For this review, use the dimensioned drawing (mm, ordinates from the lowest corner) and the shaded views. A direction names the side the tool comes from. Round coordinates to 2 decimals unless told otherwise and drop trailing zeros. Order: outer loops, then holes, each group sorted by start corner. A loop starts at its lowest first (then second) coordinate and runs counter-clockwise, first axis right, second up. Notation, with made-up numbers: (-29.5, 18.25) - (-1.5, 18.25) arc R14 ccw to (-1.5, 29.25) - close; hole circle Ø6 at (-29, 80). An arc over 180 degrees is marked (long way). Write each question's results on one line, items separated by ' | '. Start each with the question number.
(1) For the marked faces 1 and 2, list the 3-axis set-ups (+Z, -Z, +X, -X, +Y, -Y) from which the entire face can be reached by the end or side of a thin tool; tool diameter is ignored.
(2) Draft analysis for pull direction X (two halves, no side actions). For the marked faces 3, 4 and 5, state which applies: pulls with the +X half, pulls with the -X half, needs draft (parallel to the pull), parting line crosses it, or undercut.
(3) Take a section at C-C, the plane x = 482.55. Give the boundary of the cut face in (y, z), plus the area to 3 significant figures.
(4) Take a section at A-A, the plane y = 286.5. Give the boundary of the cut face in (x, z).
(5) Take a section at D-D, the plane y = 484. Give the boundary of the cut face in (x, z).
(6) Take a section at B-B, the plane z = 54. Give the boundary of the cut face in (x, y), plus the area to 3 significant figures.
(7) For L1, parallel to X at y = 526, z = 31; L2, parallel to X at y = 282.5, z = 18; L3, parallel to Y at x = 495, z = 94.5, list the stretches that pass through material, from the lowest coordinate up. Write a range as from..to.
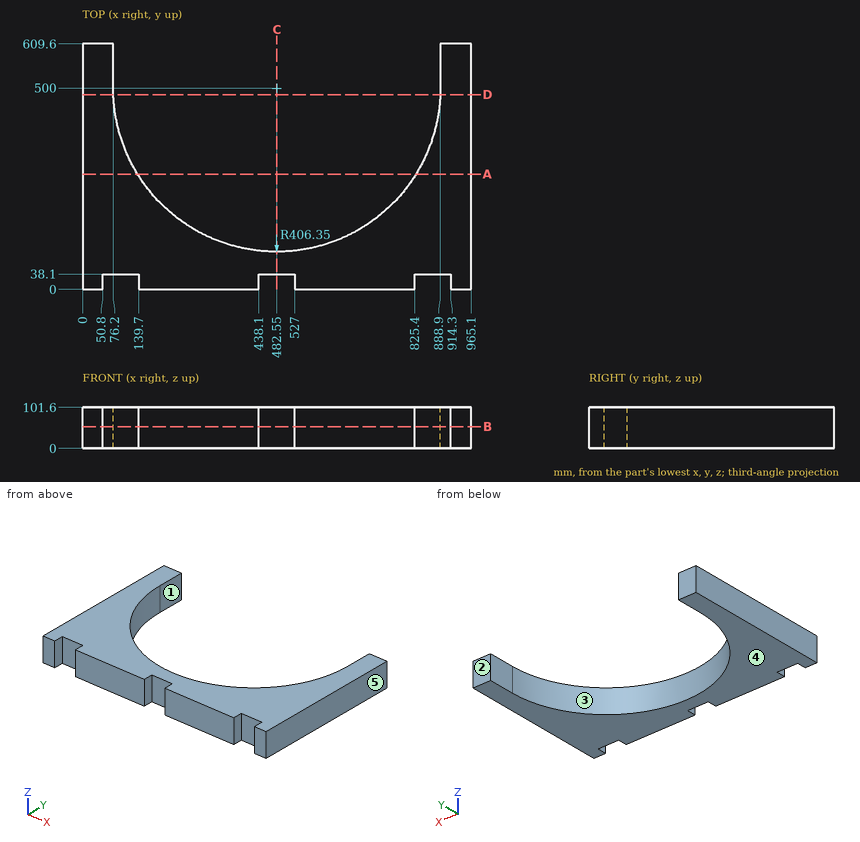
Results below:
1) face 1: +Z, -Z, +Y | face 2: +Z, -Z, +X, -X, +Y
2) face 3: undercut | face 4: needs draft | face 5: pulls with the +X half
3) outline: (38.1, 0) - (93.65, 0) - (93.65, 101.6) - (38.1, 101.6) - close | area: 5,640 mm^2
4) outline: (0, 0) - (136.81, 0) - (136.81, 101.6) - (0, 101.6) - close; (828.29, 0) - (965.1, 0) - (965.1, 101.6) - (828.29, 101.6) - close
5) outline: (0, 0) - (76.52, 0) - (76.52, 101.6) - (0, 101.6) - close; (888.58, 0) - (965.1, 0) - (965.1, 101.6) - (888.58, 101.6) - close
6) outline: (0, 0) - (50.8, 0) - (50.8, 38.1) - (139.7, 38.1) - (139.7, 0) - (438.1, 0) - (438.1, 38.1) - (527, 38.1) - (527, 0) - (825.4, 0) - (825.4, 38.1) - (914.3, 38.1) - (914.3, 0) - (965.1, 0) - (965.1, 609.6) - (888.9, 609.6) - (888.9, 500) arc R406.35 cw to (76.2, 500) - (76.2, 609.6) - (0, 609.6) - close | area: 230,000 mm^2
7) L1: x = 0..76.2, 888.9..965.1 | L2: x = 0..139.31, 825.79..965.1 | L3: y = 38.1..93.84
